from build123d import *

# Parameters (mm, degrees)
SKETCH1_R           = 75
BOSS_EXTRUDE1_DEPTH = 10
SKETCH2_R           = 16
CUT_EXTRUDE1_DEPTH  = 30
SKETCH3_R           = 2.25
CUT_EXTRUDE2_DEPTH  = 30
SKETCH4_R           = 2.25
CUT_EXTRUDE3_DEPTH  = 30
SKETCH5_R           = 2.25
CUT_EXTRUDE4_DEPTH  = 30
SKETCH6_R           = 2.25
CUT_EXTRUDE5_DEPTH  = 30


with BuildPart() as part:
    # Sketch1 → Boss-Extrude1 (new body)
    with BuildSketch(Plane.XY.offset(113)):
        with Locations((300, 300)):
            Circle(SKETCH1_R)
    extrude(amount=BOSS_EXTRUDE1_DEPTH)

    # Sketch2 → Cut-Extrude1 (cut)
    with BuildSketch(Plane.XY.offset(123)):
        with Locations((300, 300)):
            Circle(SKETCH2_R)
    extrude(amount=-CUT_EXTRUDE1_DEPTH, mode=Mode.SUBTRACT)

    # Sketch3 → Cut-Extrude2 (cut)
    with BuildSketch(Plane.XY.offset(123)):
        with Locations((345, 300)):
            Circle(SKETCH3_R)
    extrude(amount=-CUT_EXTRUDE2_DEPTH, mode=Mode.SUBTRACT)

    # Sketch4 → Cut-Extrude3 (cut)
    with BuildSketch(Plane.XY.offset(123)):
        with Locations((255, 300)):
            Circle(SKETCH4_R)
    extrude(amount=-CUT_EXTRUDE3_DEPTH, mode=Mode.SUBTRACT)

    # Sketch5 → Cut-Extrude4 (cut)
    with BuildSketch(Plane.XY.offset(123)):
        with Locations((300, 345)):
            Circle(SKETCH5_R)
    extrude(amount=-CUT_EXTRUDE4_DEPTH, mode=Mode.SUBTRACT)

    # Sketch6 → Cut-Extrude5 (cut)
    with BuildSketch(Plane.XY.offset(123)):
        with Locations((300, 255)):
            Circle(SKETCH6_R)
    extrude(amount=-CUT_EXTRUDE5_DEPTH, mode=Mode.SUBTRACT)


solid = part.part
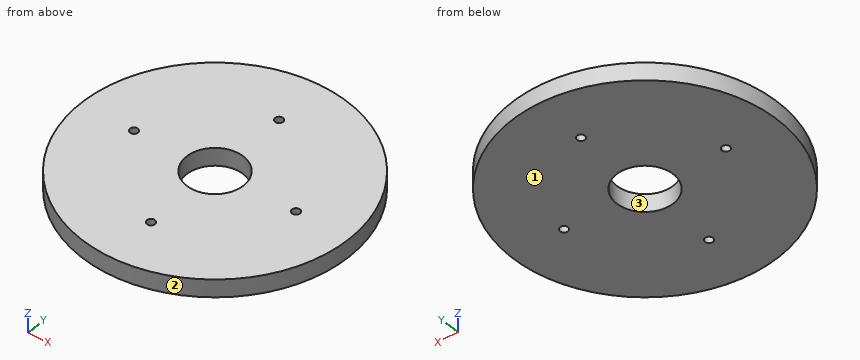
Work out the finished part from the listing and answer in its coordinate system (mm). Face numbers are marked on the shaded views. Round coordinates to 2 decimals unless told otherwise and drop trailing zeros. Write each loop counter-clockwise with the first axis right and the second up, starting at its lowest first coordinate (ties: lowest second). Pieces come first, ordered by that corner, then holes. Notation, with made-up numbers: (-26.75, -1) -> (-16.75, -1) arc R25 ccw to (-16.75, 32) -> close; hole circle Ø4 at (35.25, -37). An arc over 180 degrees is marked (long way). Write each question's results on one line, items separated by ' | '.
Item 1: A cutting plane is placed at A-A, the plane y = 345. Determine the outline of the cut face in (x, z).
Result set:
outline: (240, 113) -> (297.75, 113) -> (297.75, 123) -> (240, 123) -> close; (302.25, 113) -> (360, 113) -> (360, 123) -> (302.25, 123) -> close
Item 2: Find the intervals of material crossed by line 1 along Y through (x, z) = (300, 121); line 2 along X through (y, z) = (255, 118.25); line 3 along Y through (x, z) = (306, 122.25), in increasing order. Write a range as [from, to].
Result set:
line 1: [225, 252.75], [257.25, 284], [316, 342.75], [347.25, 375] | line 2: [240, 297.75], [302.25, 360] | line 3: [225.24, 285.17], [314.83, 374.76]
Item 3: The mould has two halves that part along X. Classify the marked faces 1, 2 and 3: +X half, -X half, draft (parallel to the pull), parting line (faces both ways), or undercut.
Result set:
face 1: draft | face 2: parting line | face 3: undercut
Item 4: Flat-ended cylindrical pins translate along their axes: P1, Ø1, axis at x = 288.5, z = 117, coming from the +Y side; P2, Ø4, axis at x = 248, z = 118.5, coming from the +Y side; P3, Ø3, axis at x = 322.5, z = 117, coming from the +Y side; P4, Ø3.5, axis at x = 255, y = 300, coming from the -Z side. Find the tip coordinate at first contact, or state that the pin passes through.
Result set:
P1: y = 374.19 | P2: y = 355.9 | P3: y = 372 | P4: through
Item 5: A cutting plane is placed at C-C, the plane x = 300. Determine the outline of the cut face in (y, z), plus the area to 3 significant figures.
Result set:
outline: (225, 113) -> (252.75, 113) -> (252.75, 123) -> (225, 123) -> close; (257.25, 113) -> (284, 113) -> (284, 123) -> (257.25, 123) -> close; (316, 113) -> (342.75, 113) -> (342.75, 123) -> (316, 123) -> close; (347.25, 113) -> (375, 113) -> (375, 123) -> (347.25, 123) -> close | area: 1,090 mm^2
